Can you work these out from the drawing? Everything is in mm from the part's minimum corner. A direction names the side the tool comes from. Give positions to 0.01 mm unless a question says otherwise; leave off trailing zeros. Write each loop counter-clockwise with the first axis right and the second up, starting at its lowest first coordinate (ties: lowest second). Pieces come first, ordered by that corner, then holes. Notation, with made-up numbers: (-29.5, 32.5) - (12.5, 32.5) arc R15 cw to (12.5, 56.5) - close; hole circle Ø10 at (-29, 39.25). An arc over 180 degrees is marked (long way). Answer in a Markdown table with one row per item.
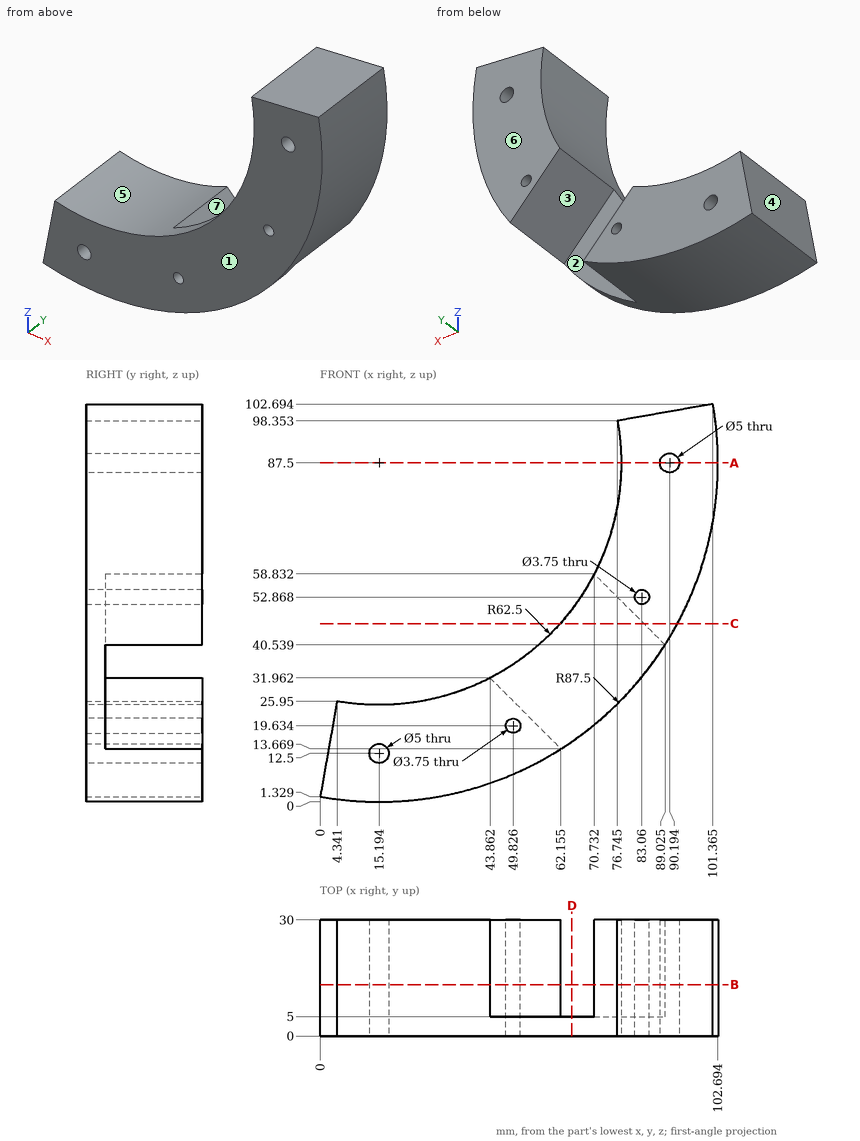
1) Imagine slicing it at C-C (z = 46). List the corners of the cut face in (x, y) for me (1 decimal).
Check values:
| item | result |
|---|---|
| outline | (61.9, 0) - (92.2, 0) - (92.2, 30) - (83.6, 30) - (83.6, 5) - (61.9, 5) - close |
2) On a 3-axis mill with a long thin cutter (end or side, diameter ignored), from which of +Z, -Z, +X, -X, +Y, -Y can I reach the whole of each face in a straight line? I mean the marked faces 1, 2 and 3. Say none if no direction works.
Check values:
| item | result |
|---|---|
| face 1 | +Z, -Z, +X, -X, -Y |
| face 2 | +Y |
| face 3 | -Z, -X, +Y |
3) If I drill on line 1 (X direction, y = 19.25, z = 87.5) (1 decimal); line 2 (Z direction, x = 88, y = 24.5) (1 decimal); line 3 (Y direction, x = 68, z = 50), over which ranges is the centre line in solid material (lowest first)?
Check values:
| item | result |
|---|---|
| line 1 | x = 77.7 to 87.7, 92.7 to 102.7 |
| line 2 | z = 41.6 to 86.3, 88.7 to 100.3 |
| line 3 | y = 0 to 5 |
4) Imagine slicing it at B-B (y = 13.25). State how many separate pieces and enclosed holes the cut face has, then the cut area to 3 significant figures.
Check values:
| item | result |
|---|---|
| separate pieces | 2 |
| enclosed holes | 4 |
| area | 2,580 mm2 |
5) Will these pins go through, and if not, where does the flat tip stop? P1, Ø3, axis at x = 90.19, z = 87.5, coming from the +Y side; P2, Ø1, axis at x = 60.5, z = 38.5, coming from the +Y side; P3, Ø10, axis at y = 4, z = 71.5, coming from the -X side.
Check values:
| item | result |
|---|---|
| P1 | passes through |
| P2 | stops at y = 5 |
| P3 | stops at x = 74.06 |
6) Imagine slicing it at A-A (z = 87.5). List the corners of the cut face in (x, y) for me (1 decimal).
Check values:
| item | result |
|---|---|
| outline | (77.7, 0) - (87.7, 0) - (87.7, 30) - (77.7, 30) - close; (92.7, 0) - (102.7, 0) - (102.7, 30) - (92.7, 30) - close |
7) Imagine slicing it at D-D (x = 65). List the corners of the cut face in (y, z) for me, then the cut area to 3 significant figures.
Check values:
| item | result |
|---|---|
| outline | (0, 15.56) - (5, 15.56) - (5, 49.74) - (0, 49.74) - close |
| area | 171 mm2 |
8) We'd pull the mould along X, two halves only. Please class the marked faces 4, 5, 6 and 7: +X half, -X half, draft (parallel to the pull), parting line (faces both ways), or undercut.
Check values:
| item | result |
|---|---|
| face 4 | -X half |
| face 5 | undercut |
| face 6 | draft |
| face 7 | +X half |
